```python
from build123d import *

# Parameters (mm, degrees)
SKETCH1_R           = 40
BOSS_EXTRUDE1_DEPTH = 10
SKETCH2_R           = 3
CUT_EXTRUDE1_DEPTH  = 195.477983176
SKETCH3_R           = 3
CUT_EXTRUDE2_DEPTH  = 195.477983176
SKETCH4_R           = 3
CUT_EXTRUDE3_DEPTH  = 195.477983176
SKETCH5_R           = 3
CUT_EXTRUDE4_DEPTH  = 195.477983176
SKETCH6_R           = 26
BOSS_EXTRUDE2_DEPTH = 16
SKETCH7_R           = 26
BOSS_EXTRUDE3_DEPTH = 6
BOSS_EXTRUDE3_TAPER = 45
SKETCH8_R           = 20
BOSS_EXTRUDE4_DEPTH = 14
SKETCH9_R           = 25.75
CUT_EXTRUDE5_DEPTH  = 10.2
SKETCH10_R          = 20
CUT_EXTRUDE6_DEPTH  = 198.492597178


with BuildPart() as part:
    # Sketch1 → Boss-Extrude1 (new body)
    with BuildSketch(Plane.XZ.offset(-11.5)):
        with Locations(Location((-150.057059695, 0, 0), (0, 0, 90))):
            Circle(SKETCH1_R)
    extrude(amount=-BOSS_EXTRUDE1_DEPTH)

    # Sketch2 → Cut-Extrude1 (cut, through all)
    with BuildSketch(Plane.XZ.offset(-11.5)):
        with Locations(Location((-150.057059695, -33.5, 0), (0, 0, 90))):
            Circle(SKETCH2_R)
    extrude(amount=-CUT_EXTRUDE1_DEPTH, mode=Mode.SUBTRACT)

    # Sketch3 → Cut-Extrude2 (cut, through all)
    with BuildSketch(Plane.XZ.offset(-11.5)):
        with Locations(Location((-116.557059695, 0, 0), (0, 0, 90))):
            Circle(SKETCH3_R)
    extrude(amount=-CUT_EXTRUDE2_DEPTH, mode=Mode.SUBTRACT)

    # Sketch4 → Cut-Extrude3 (cut, through all)
    with BuildSketch(Plane.XZ.offset(-11.5)):
        with Locations(Location((-150.057059695, 33.5, 0), (0, 0, 90))):
            Circle(SKETCH4_R)
    extrude(amount=-CUT_EXTRUDE3_DEPTH, mode=Mode.SUBTRACT)

    # Sketch5 → Cut-Extrude4 (cut, through all)
    with BuildSketch(Plane(origin=(0, 21.5, 0), x_dir=(-1, 0, 0), z_dir=(0, 1, 0))):
        with Locations(Location((183.557059695, 0, 0), (0, 0, 270))):
            Circle(SKETCH5_R)
    extrude(amount=-CUT_EXTRUDE4_DEPTH, mode=Mode.SUBTRACT)

    # Sketch6 → Boss-Extrude2 (add)
    with BuildSketch(Plane(origin=(0, 21.5, 0), x_dir=(-1, 0, 0), z_dir=(0, 1, 0))):
        with Locations(Location((150.057059695, 0, 0), (0, 0, 90))):
            Circle(SKETCH6_R)
    extrude(amount=BOSS_EXTRUDE2_DEPTH)

    # Sketch7 → Boss-Extrude3 (add)
    with BuildSketch(Plane(origin=(0, 37.5, 0), x_dir=(-1, 0, 0), z_dir=(0, 1, 0))):
        with Locations(Location((150.057059695, 0, 0), (0, 0, 90))):
            Circle(SKETCH7_R)
    extrude(amount=BOSS_EXTRUDE3_DEPTH, taper=BOSS_EXTRUDE3_TAPER)

    # Sketch8 → Boss-Extrude4 (add)
    with BuildSketch(Plane(origin=(0, 43.5, 0), x_dir=(-1, 0, 0), z_dir=(0, 1, 0))):
        with Locations(Location((150.057059695, 0, 0), (0, 0, 90))):
            Circle(SKETCH8_R)
    extrude(amount=BOSS_EXTRUDE4_DEPTH)

    # Sketch9 → Cut-Extrude5 (cut)
    with BuildSketch(Plane.XZ.offset(-11.5)):
        with Locations(Location((-150.057059695, 0, 0), (0, 0, 90))):
            Circle(SKETCH9_R)
    extrude(amount=-CUT_EXTRUDE5_DEPTH, mode=Mode.SUBTRACT)

    # Sketch10 → Cut-Extrude6 (cut, through all)
    with BuildSketch(Plane.XZ.offset(-21.7)):
        with Locations(Location((-150.057059695, 0, 0), (0, 0, 270))):
            Circle(SKETCH10_R)
    extrude(amount=-CUT_EXTRUDE6_DEPTH, mode=Mode.SUBTRACT)


solid = part.part
```
Could you check a few things on this model? Use its own coordinates, in mm. A direction names the side the tool comes from. Give positions to 0.01 mm unless a question says otherwise; leave off trailing zeros. Loops run counter-clockwise (first coordinate to the right, second up) from the corner with the lowest first, then second, coordinate; pieces in that order, holes last. Notation, with made-up numbers: (-14, 79) -> (-8, 79) arc R8 ccw to (-8, 93) -> close; hole circle Ø6 at (73.25, 68). An arc over 180 degrees is marked (long way). Put each result on its own line as item: value.
(1) For faces 4 (the face through (-142, 21.5, 26)), 5 (the face through (-147.13, 16.43, -34.15)), 6 (the face through (-175.59, 16.53, -3.35)), which set-ups out of +Z, -Z, +X, -X, +Y, -Y let a thin tool reach every point of the face, with its end or its side?
Computed:
face 4: +Y
face 5: +Y, -Y
face 6: -Y
(2) Imagine slicing it at D-D on y = 39.5. Write out the boundary of the cut face in (x, z), plus the area to 3 significant figures.
Computed:
outline: circle Ø48 at (-150.06, 0); hole circle Ø40 at (-150.06, 0)
area: 553 mm^2
(3) Imagine slicing it at B-B on x = -118. Write out the boundary of the cut face in (y, z), plus the area to 3 significant figures.
Computed:
outline: (11.5, -23.92) -> (21.5, -23.92) -> (21.5, -2.63) -> (11.5, -2.63) -> close; (11.5, 2.63) -> (21.5, 2.63) -> (21.5, 23.92) -> (11.5, 23.92) -> close
area: 426 mm^2
(4) Please list where these lines run through material, in increasing order: probe 1 along X at (y, z) = (13, 0); probe 2 along X at (y, z) = (36.5, 0); probe 3 along X at (y, z) = (41, 14.5). Write a range as [from, to].
Computed:
probe 1: [-190.06, -186.56], [-180.56, -175.81], [-124.31, -119.56], [-113.56, -110.06]
probe 2: [-176.06, -170.06], [-130.06, -124.06]
probe 3: [-167.26, -163.83], [-136.28, -132.85]
(5) I'm going to push flat-ended pins straight in: pin 1 Ø3 at (x, y) = (-124, 18.5) entering from +Z; pin 2 Ø1.5 at (x, y) = (-156.5, 34) entering from +Z; pin 3 Ø5 at (x, z) = (-116.56, 0) entering from -Y; pin 4 Ø10 at (x, z) = (-148, 15) entering from -Y. Where does each tip first touch, or does it pass through?
Computed:
pin 1: z = 31.57
pin 2: z = 25.37
pin 3: through
pin 4: y = 21.7
(6) Imagine slicing it at A-A on z = 0. Write out the boundary of the cut face in (x, y), plus the area to 3 significant figures.
Computed:
outline: (-190.06, 11.5) -> (-186.56, 11.5) -> (-186.56, 21.5) -> (-190.06, 21.5) -> close; (-180.56, 11.5) -> (-175.81, 11.5) -> (-175.81, 21.7) -> (-170.06, 21.7) -> (-170.06, 43.5) -> (-176.06, 37.5) -> (-176.06, 21.5) -> (-180.56, 21.5) -> close; (-130.06, 21.7) -> (-124.31, 21.7) -> (-124.31, 11.5) -> (-119.56, 11.5) -> (-119.56, 21.5) -> (-124.06, 21.5) -> (-124.06, 37.5) -> (-130.06, 43.5) -> close; (-113.56, 11.5) -> (-110.06, 11.5) -> (-110.06, 21.5) -> (-113.56, 21.5) -> close
area: 391 mm^2
(7) Thinking about a two-plate mould opening in X: for faces 1 (the face through (-180.896, 16.57, -1.384)), 2 (the face through (-124, 11.5, -1)), 3 (the face through (-111.01, 16.43, -8.67)), which applies, pulls with the +X half, pulls with the -X half, needs draft (parallel to the pull), parting line crosses it, or undercut?
Computed:
face 1: undercut
face 2: needs draft
face 3: parting line crosses it
(8) Imagine slicing it at C-C on z = -31.5. Write out the boundary of the cut face in (x, y), plus the area to 3 significant figures.
Computed:
outline: (-174.71, 11.5) -> (-152.29, 11.5) -> (-152.29, 21.5) -> (-174.71, 21.5) -> close; (-147.82, 11.5) -> (-125.4, 11.5) -> (-125.4, 21.5) -> (-147.82, 21.5) -> close
area: 448 mm^2
